from build123d import *

# Parameters (mm, degrees)
SKETCH_1_R      = 2.75
EXTRUDE_1_DEPTH = 2


with BuildPart() as part:
    # 草图1 → 凸台-拉伸1 (new body)
    with BuildSketch(Plane(origin=(0, 0, 0), x_dir=(1, 0, 0), z_dir=(0, 1, 0))):
        Polygon((0, 0), (90, 0), (90, -20), (20, -20), (20, -60), (0, -60), align=None)
        with Locations(Location((10, -54, 0), (0, 0, 270))):
            Circle(SKETCH_1_R, mode=Mode.SUBTRACT)
        with Locations(Location((82, -10, 0), (0, 0, 270))):
            Circle(SKETCH_1_R, mode=Mode.SUBTRACT)
        with Locations(Location((10, -43, 0), (0, 0, 270))):
            Circle(SKETCH_1_R, mode=Mode.SUBTRACT)
        with Locations(Location((10, -32, 0), (0, 0, 270))):
            Circle(SKETCH_1_R, mode=Mode.SUBTRACT)
        with Locations(Location((71, -10, 0), (0, 0, 270))):
            Circle(SKETCH_1_R, mode=Mode.SUBTRACT)
        with Locations(Location((60, -10, 0), (0, 0, 270))):
            Circle(SKETCH_1_R, mode=Mode.SUBTRACT)
        with Locations(Location((10, -10, 0), (0, 0, 270))):
            Circle(SKETCH_1_R, mode=Mode.SUBTRACT)
    extrude(amount=EXTRUDE_1_DEPTH)


solid = part.part
Geometry check sheet. Reference: the model listing, model coordinates, mm. A direction names the side the tool comes from. Give positions to 0.01 mm unless a question says otherwise; leave off trailing zeros. Write each loop counter-clockwise with the first axis right and the second up, starting at its lowest first coordinate (ties: lowest second). Pieces come first, ordered by that corner, then holes.
1) Cross-section at C-C (x = 10). Record the boundary of the cut face in (y, z), plus the area to 3 significant figures.
Values follow:
outline: (0, 0) - (2, 0) - (2, 7.25) - (0, 7.25) - close; (0, 12.75) - (2, 12.75) - (2, 29.25) - (0, 29.25) - close; (0, 34.75) - (2, 34.75) - (2, 40.25) - (0, 40.25) - close; (0, 45.75) - (2, 45.75) - (2, 51.25) - (0, 51.25) - close; (0, 56.75) - (2, 56.75) - (2, 60) - (0, 60) - close
area: 76.0 mm2
2) Cross-section at B-B (z = 10). Record the boundary of the cut face in (x, y).
Values follow:
outline: (0, 0) - (7.25, 0) - (7.25, 2) - (0, 2) - close; (12.75, 0) - (57.25, 0) - (57.25, 2) - (12.75, 2) - close; (62.75, 0) - (68.25, 0) - (68.25, 2) - (62.75, 2) - close; (73.75, 0) - (79.25, 0) - (79.25, 2) - (73.75, 2) - close; (84.75, 0) - (90, 0) - (90, 2) - (84.75, 2) - close
3) Cross-section at A-A (x = 82). Record the boundary of the cut face in (y, z), plus the area to 3 significant figures.
Values follow:
outline: (0, 0) - (2, 0) - (2, 7.25) - (0, 7.25) - close; (0, 12.75) - (2, 12.75) - (2, 20) - (0, 20) - close
area: 29.0 mm2
4) Release check for a two-part mould opening along Z. For faces 3 (the face through (90, 1, 10)), 4 (the face through (82.83, 0.99, 12.62)), 5 (the face through (10, 1, 60)) record: released by +Z, released by -Z, zero draft, split by the parting line, or undercut.
Values follow:
face 3: zero draft
face 4: undercut
face 5: released by +Z
5) Thickness scan on line 1 (X direction, y = 0.6, z = 10); line 2 (X direction, y = 1.15, z = 54); line 3 (Z direction, x = 47, y = 1.9). Record the ranges inside material, lowest first.
Values follow:
line 1: x = 0 to 7.25, 12.75 to 57.25, 62.75 to 68.25, 73.75 to 79.25, 84.75 to 90
line 2: x = 0 to 7.25, 12.75 to 20
line 3: z = 0 to 20
6) Cross-section at D-D (y = 0.9). Record the boundary of the cut face in (x, z), plus the area to 3 significant figures.
Values follow:
outline: (0, 0) - (90, 0) - (90, 20) - (20, 20) - (20, 60) - (0, 60) - close; hole circle Ø5.5 at (10, 10); hole circle Ø5.5 at (10, 32); hole circle Ø5.5 at (10, 43); hole circle Ø5.5 at (10, 54); hole circle Ø5.5 at (60, 10); hole circle Ø5.5 at (71, 10); hole circle Ø5.5 at (82, 10)
area: 2,430 mm2
7) Set-up check for faces 1 (the face through (20, 1, 40)), 2 (the face through (10.121, 0.986, 51.253)): record each of +Z, -Z, +X, -X, +Y, -Y from which the full face is reachable in a straight line by a thin tool's end or side.
Values follow:
face 1: +Z, +X, +Y, -Y
face 2: +Y, -Y
8) Go/stop test with a flat-tipped pin: pin 1 Ø1 at (y, z) = (1, 47) entering from +X. Record where the tip stops, or that it passes through.
Values follow:
pin 1: stops at x = 20
